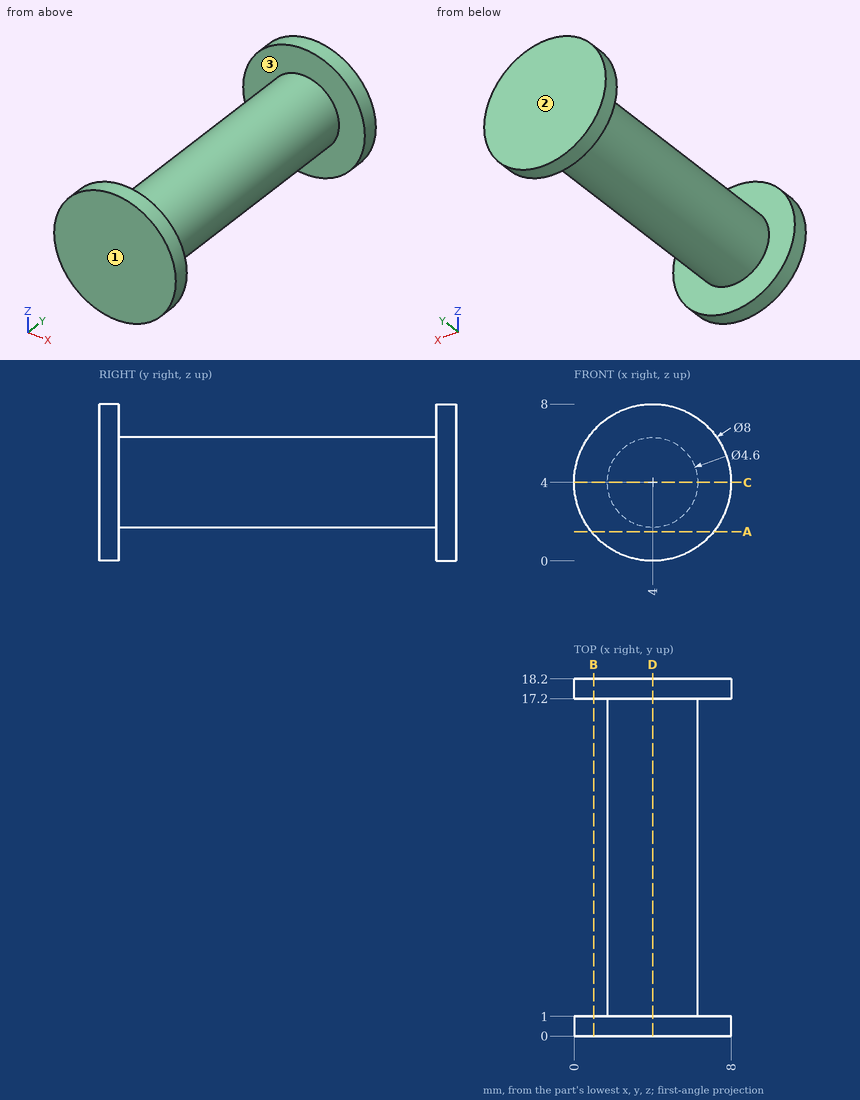
Geometry check sheet. Reference: drawing and pictorial views, mm from the part's lowest x, y, z. Round coordinates to 2 decimals unless told otherwise and drop trailing zeros. Loops run counter-clockwise (first coordinate to the right, second up) from the corner with the lowest first, then second, coordinate; pieces in that order, holes last. Notation, with made-up numbers: (-5, -1) - (35, -1) arc R17 ccw to (35, 26) - close; hole circle Ø5 at (66, 22.25). An arc over 180 degrees is marked (long way). Answer in a Markdown table with one row per item. Add a question column.
Q1. Section check A-A on z = 1.5. Enter the section's corners in (x, y).
Q2. Gauge pin test, flat ends, axial feed: pin 1 (3 mm diameter, centred on y = 9.5, z = 1.5, fed in from -X); pin 2 (1.5 mm diameter, centred on y = 16, z = 2, fed in from -X); pin 3 (1.5 mm diameter, centred on x = 1.5, y = 15.5, fed in from +Z). Record the tip position at first contact, or that the pin passes through.
Q3. Section check D-D on x = 4. Enter the section's corners in (y, z).
Q4. Material ranges on line 1 (Y direction, x = 5.5, z = 6.5); line 2 (Z direction, x = 2.75, y = 8.75); line 3 (Z direction, x = 4.25, y = 13.25), recorded low to high.
Q5. Section check B-B on x = 1. Enter the section's corners in (y, z).
Q6. Section check C-C on z = 4. Enter the section's corners in (x, y), plus the area to 3 significant figures.
Q7. Release check for a two-part mould opening along Y. For the marked faces 1, 2 and 3 record: pulls with the +Y half, pulls with the -Y half, needs draft (parallel to the pull), parting line crosses it, or undercut.
Found:
| question | item | result |
|---|---|---|
| 1 | outline | (0.88, 0) - (7.12, 0) - (7.12, 1) - (0.88, 1) - close; (0.88, 17.2) - (7.12, 17.2) - (7.12, 18.2) - (0.88, 18.2) - close |
| 2 | pin 1 | stops at x = 1.93 |
| 2 | pin 2 | stops at x = 2.07 |
| 2 | pin 3 | stops at z = 5.49 |
| 3 | outline | (0, 0) - (1, 0) - (1, 1.7) - (17.2, 1.7) - (17.2, 0) - (18.2, 0) - (18.2, 8) - (17.2, 8) - (17.2, 6.3) - (1, 6.3) - (1, 8) - (0, 8) - close |
| 4 | line 1 | y = 0 to 1, 17.2 to 18.2 |
| 4 | line 2 | z = 2.07 to 5.93 |
| 4 | line 3 | z = 1.71 to 6.29 |
| 5 | outline | (0, 1.35) - (1, 1.35) - (1, 6.65) - (0, 6.65) - close; (17.2, 1.35) - (18.2, 1.35) - (18.2, 6.65) - (17.2, 6.65) - close |
| 6 | outline | (0, 0) - (8, 0) - (8, 1) - (6.3, 1) - (6.3, 17.2) - (8, 17.2) - (8, 18.2) - (0, 18.2) - (0, 17.2) - (1.7, 17.2) - (1.7, 1) - (0, 1) - close |
| 6 | area | 90.5 mm² |
| 7 | face 1 | pulls with the -Y half |
| 7 | face 2 | pulls with the +Y half |
| 7 | face 3 | undercut |
